Part print with two shaded views. Sizes in mm from the minimum x, y, z corner. A direction names the side the tool comes from. Round coordinates to 2 decimals unless told otherwise and drop trailing zeros. Loops run counter-clockwise (first coordinate to the right, second up) from the corner with the lowest first, then second, coordinate; pieces in that order, holes last. Notation, with made-up numbers: (3, 75.5) - (37, 75.5) arc R23 cw to (37, 113.5) - close; hole circle Ø6 at (84, 40). An arc over 180 degrees is marked (long way). Put each result on its own line as item: value. Start each with the question number.
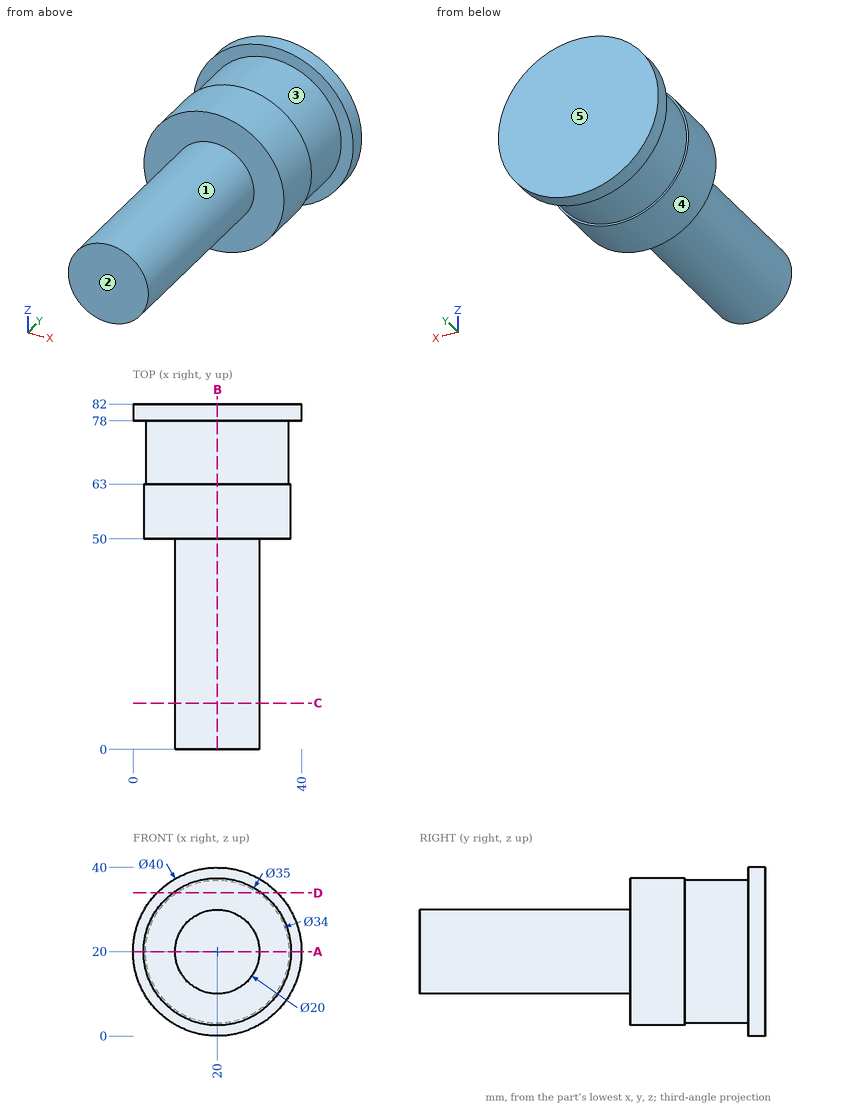
1) Which spindle directions (+Z, -Z, +X, -X, +Y, -Y) get a long thin tool onto all of the face, cutting with end or side? Do the marked faces 1 and 2. Say none if no direction does.
2) Slice it at A-A, the plane z = 20. Write the cut outline in (x, y), and give its area (4 significant figures).
3) Slice it at D-D, the plane z = 34. Write the cut outline in (x, y).
4) Slice it at C-C, the plane y = 11. Write the cut outline in (x, z), and give its area (3 significant figures).
5) Drill centre lines: line 1 (Y direction, x = 30, z = 16.5); line 2 (X direction, y = 76, z = 20.5); line 3 (X direction, y = 62.5, z = 34). Where is each one in solid material? Low to high. Write a range as [from, to].
6) Slice it at B-B, the plane x = 20. Write the cut outline in (y, z).
7) Drop flat-ended pins along their axis: pin 1 Ø8 at (y, z) = (63, 34) entering from +X; pin 2 Ø5 at (x, z) = (18.5, 33) entering from -Y; pin 3 Ø12 at (y, z) = (72.5, 16) entering from +X; pin 4 Ø1.5 at (x, y) = (7.5, 28) entering from -Z. Give the stop position or say it passes through.
8) Pull direction Y, two halves, no side cores. Call the marked faces 3, 4 and 5: pulls with the +Y half, pulls with the -Y half, needs draft (parallel to the pull), parting line crosses it, or undercut.
Taken from the geometry:
1. face 1: -Y
1. face 2: +Z, -Z, +X, -X, -Y
2. outline: (0, 78) - (3, 78) - (3, 63) - (2.5, 63) - (2.5, 50) - (10, 50) - (10, 0) - (30, 0) - (30, 50) - (37.5, 50) - (37.5, 63) - (37, 63) - (37, 78) - (40, 78) - (40, 82) - (0, 82) - close
2. area: 2,125 mm2
3. outline: (5.72, 78) - (10.36, 78) - (10.36, 63) - (9.5, 63) - (9.5, 50) - (30.5, 50) - (30.5, 63) - (29.64, 63) - (29.64, 78) - (34.28, 78) - (34.28, 82) - (5.72, 82) - close
4. outline: circle Ø20 at (20, 20)
4. area: 314 mm2
5. line 1: y = [50, 82]
5. line 2: x = [3.01, 36.99]
5. line 3: x = [9.5, 30.5]
6. outline: (0, 10) - (50, 10) - (50, 2.5) - (63, 2.5) - (63, 3) - (78, 3) - (78, 0) - (82, 0) - (82, 40) - (78, 40) - (78, 37) - (63, 37) - (63, 37.5) - (50, 37.5) - (50, 30) - (0, 30) - close
7. pin 1: stops at x = 34.36
7. pin 2: stops at y = 50
7. pin 3: stops at x = 39.94
7. pin 4: passes through
8. face 3: undercut
8. face 4: needs draft
8. face 5: pulls with the +Y half
